from build123d import *

# Parameters (mm, degrees)
F2_R     = 9.525
F3_DEPTH = 88.9


with BuildPart() as f1:
    # F0 (on Front) → F1 (revolve)
    with BuildSketch(Plane.XZ):
        Polygon((-16.631375, -91.427677), (2.418625, -91.427677), (2.418625, -2.527677), (-42.031375, -2.527677), (-42.031375, -21.577677), (-22.981375, -21.577677), (-22.981375, -78.727677), (-16.631375, -78.727677), align=None)
    revolve(axis=Axis((2.418625, 0, 3.463581), (0, 0, 1)))

    # F2 (on face) → F3 (cut)
    with BuildSketch(Plane(origin=(0, 0, -91.427677), x_dir=(1, 0, 0), z_dir=(0, 0, -1))):
        with Locations((2.418625, 0)):
            Circle(F2_R)
    extrude(amount=-F3_DEPTH, mode=Mode.SUBTRACT)


solid = f1.part
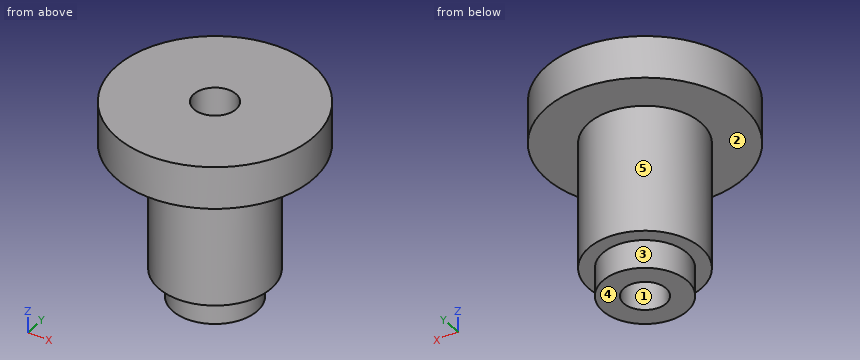
Geometry: final body of the model. Coordinates: model frame, mm. Face numbers are marked on the shaded views. A direction names the side the tool comes from. Give positions to 0.01 mm unless a question says otherwise; leave off trailing zeros. Order: outer loops, then holes, each group sorted by start corner. A loop starts at its lowest first (then second) coordinate and runs counter-clockwise, first axis right, second up. Notation, with made-up numbers: (36.25, -22.75) -> (81.25, -22.75) arc R13 cw to (81.25, -18.75) -> close; hole circle Ø3 at (25, -37.5). An arc over 180 degrees is marked (long way). Write each question's results on one line, items separated by ' | '.
1) Cut plane D-D (y = -15.5). Output: boundary loops of the cut face in (x, z), and give its area (3 significant figures).
Geometry says:
outline: (-39.24, -21.58) -> (-17.7, -21.58) -> (-17.7, -78.73) -> (-8.66, -78.73) -> (-8.66, -91.43) -> (13.49, -91.43) -> (13.49, -78.73) -> (22.54, -78.73) -> (22.54, -21.58) -> (44.08, -21.58) -> (44.08, -2.53) -> (-39.24, -2.53) -> close | area: 4,170 mm²
2) Line query: line 1 along X through (y, z) = (0, -50); line 2 along Z through (x, y) = (33, -0.5); line 3 along Y through (x, z) = (-28, -17). Output: solid intervals per line, ascending.
Geometry says:
line 1: x = -22.98 to -7.11, 11.94 to 27.82 | line 2: z = -21.58 to -2.53 | line 3: y = -32.41 to 32.41
3) Set-up query: the marked faces 4 and 5. Return all of +Z, -Z, +X, -X, +Y, -Y with unobstructed straight access to the full face (end or side cutting, diameter ignored); none if empty.
Geometry says:
face 4: -Z, +X, -X, +Y, -Y | face 5: -Z
4) Cut plane C-C (z = -24). Output: boundary loops of the cut face in (x, y) (3 decimals).
Geometry says:
outline: circle Ø50.8 at (2.419, 0); hole circle Ø19.05 at (2.419, 0)
5) Draft query along Y for the marked faces 1, 2 and 3. Return one class per face: released by +Y, released by -Y, zero draft, split by the parting line, or undercut.
Geometry says:
face 1: undercut | face 2: zero draft | face 3: split by the parting line
6) Cut plane A-A (y = 0). Output: boundary loops of the cut face in (x, z).
Geometry says:
outline: (-42.03, -21.58) -> (-22.98, -21.58) -> (-22.98, -78.73) -> (-16.63, -78.73) -> (-16.63, -91.43) -> (-7.11, -91.43) -> (-7.11, -2.53) -> (-42.03, -2.53) -> close; (11.94, -91.43) -> (21.47, -91.43) -> (21.47, -78.73) -> (27.82, -78.73) -> (27.82, -21.58) -> (46.87, -21.58) -> (46.87, -2.53) -> (11.94, -2.53) -> close
7) First-contact query: pin 1 Ø4 at (x, y) = (-7.5, -27.5) entering from -Z; pin 2 Ø4 at (x, z) = (-7, -81) entering from +Y; pin 3 Ø12 at (x, z) = (23.5, -40) entering from +Y. Flat tips, straight axial feed; report the tip coordinate or a pass-through.
Geometry says:
pin 1: stops at z = -21.58 | pin 2: stops at y = 17.55 | pin 3: stops at y = 20.44
8) Cut plane B-B (x = -4.5). Output: boundary loops of the cut face in (y, z).
Geometry says:
outline: (-43.91, -21.58) -> (-24.44, -21.58) -> (-24.44, -78.73) -> (-17.75, -78.73) -> (-17.75, -91.43) -> (-6.55, -91.43) -> (-6.55, -2.53) -> (-43.91, -2.53) -> close; (6.55, -91.43) -> (17.75, -91.43) -> (17.75, -78.73) -> (24.44, -78.73) -> (24.44, -21.58) -> (43.91, -21.58) -> (43.91, -2.53) -> (6.55, -2.53) -> close
